Check sheet for the modelled part. Datum: model origin and axes. Units: mm. Face numbers are marked on the shaded views. A direction names the side the tool comes from. Round coordinates to 2 decimals unless told otherwise and drop trailing zeros. Order: outer loops, then holes, each group sorted by start corner. A loop starts at its lowest first (then second) coordinate and runs counter-clockwise, first axis right, second up. Notation, with made-up numbers: (-8.75, 69.25) -> (29.25, 69.25) arc R19 ccw to (29.25, 74.25) -> close; hole circle Ø2 at (83, 82.25). An arc over 180 degrees is marked (long way). Use CSV: the item, a comma, the result in double quotes.
```python
from build123d import *

# Parameters (mm, degrees)
MODEL_R             = 1.25
BOSS_EXTRUDE1_DEPTH = 2


with BuildPart() as part:
    # Model → Boss-Extrude1 (new body)
    with BuildSketch(Plane.XY):
        with BuildLine():
            Line((1953.676808721, 1458.884115951), (1951.176808721, 1458.884115951))
            Line((1951.176808721, 1458.884115951), (1951.176808721, 1462.134115951))
            ThreePointArc((1951.176808721, 1462.134115951), (1956.676808721, 1464.884115951), (1962.176808721, 1462.134115951))
            Line((1962.176808721, 1462.134115951), (1962.176808721, 1458.884115951))
            Line((1962.176808721, 1458.884115951), (1959.676808721, 1458.884115951))
            Line((1959.676808721, 1458.884115951), (1959.676808721, 1456.884115951))
            Line((1959.676808721, 1456.884115951), (1953.676808721, 1456.884115951))
            Line((1953.676808721, 1456.884115951), (1953.676808721, 1458.884115951))
        make_face()
        with Locations((1959.176808721, 1460.884115951)):
            Circle(MODEL_R, mode=Mode.SUBTRACT)
        with Locations((1954.176808721, 1460.884115951)):
            Circle(MODEL_R, mode=Mode.SUBTRACT)
    extrude(amount=BOSS_EXTRUDE1_DEPTH)


solid = part.part
```
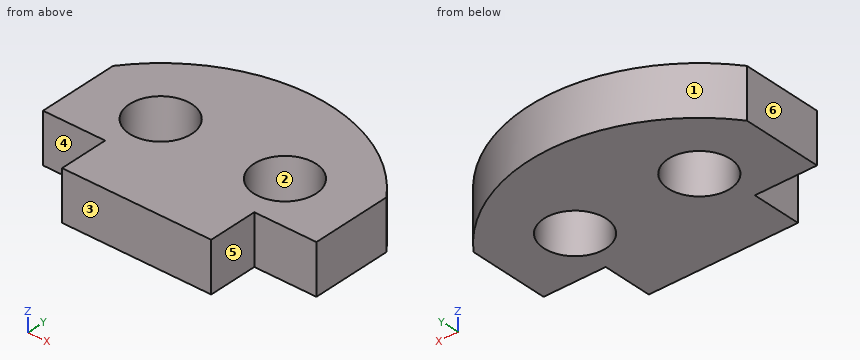
Q1. Go/stop test with flat-tipped pins: pin 1 (1.5 mm diameter, centred on x = 1954.18, y = 1460.88, fed in from +Z); pin 2 (0.6 mm diameter, centred on x = 1952, z = 0.5, fed in from -Y); pin 3 (1 mm diameter, centred on y = 1458, z = 1, fed in from -X). Record where each tip stops, or that it passes through.
Result sheet:
pin 1,"passes through"
pin 2,"stops at y = 1458.88"
pin 3,"stops at x = 1953.68"
Q2. Sectioned sample at C-C, the plane z = 1. Enter the section's corners in (x, y) (3 decimals).
Result sheet:
outline,"(1951.177, 1458.884) -> (1953.677, 1458.884) -> (1953.677, 1456.884) -> (1959.677, 1456.884) -> (1959.677, 1458.884) -> (1962.177, 1458.884) -> (1962.177, 1462.134) arc R6.875 ccw to (1951.177, 1462.134) -> close; hole circle Ø2.5 at (1954.177, 1460.884); hole circle Ø2.5 at (1959.177, 1460.884)"
Q3. Mould release check, pull along Y, two halves, no side actions. Record for the marked faces 1, 2 and 3: pulls with the +Y half, pulls with the -Y half, needs draft (parallel to the pull), parting line crosses it, or undercut.
Result sheet:
face 1,"pulls with the +Y half"
face 2,"undercut"
face 3,"pulls with the -Y half"
Q4. Sectioned sample at B-B, the plane y = 1462. Enter the section's corners in (x, z).
Result sheet:
outline,"(1951.18, 0) -> (1953.61, 0) -> (1953.61, 2) -> (1951.18, 2) -> close; (1954.74, 0) -> (1958.61, 0) -> (1958.61, 2) -> (1954.74, 2) -> close; (1959.74, 0) -> (1962.18, 0) -> (1962.18, 2) -> (1959.74, 2) -> close"
Q5. Sectioned sample at D-D, the plane y = 1458. Enter the section's corners in (x, z), then the cut area to 3 significant figures.
Result sheet:
outline,"(1953.68, 0) -> (1959.68, 0) -> (1959.68, 2) -> (1953.68, 2) -> close"
area,"12.0 mm^2"
Q6. Scan lines: L1, parallel to X at y = 1460, z = 0.65; L2, parallel to X at y = 1460.25, z = 1.3; L3, parallel to Y at x = 1954, z = 1.35. Record each from-to range of solid material in increasing order.
Result sheet:
L1,"x = 1951.18 to 1953.29, 1955.06 to 1958.29, 1960.06 to 1962.18"
L2,"x = 1951.18 to 1953.1, 1955.25 to 1958.1, 1960.25 to 1962.18"
L3,"y = 1456.88 to 1459.65, 1462.12 to 1464.34"
Q7. Access from +Z, -Z, +X, -X, +Y, -Y to the whole of each face (thin tool, end or side, straight path). Record for the marked faces 4, 5 and 6.
Result sheet:
face 4,"+Z, -Z, -X, -Y"
face 5,"+Z, -Z, +X, -Y"
face 6,"+Z, -Z, -X, +Y, -Y"
Q8. Sectioned sample at A-A, the plane x = 1954.5. Enter the section's corners in (y, z), then the cut area to 3 significant figures.
Result sheet:
outline,"(1456.88, 0) -> (1459.68, 0) -> (1459.68, 2) -> (1456.88, 2) -> close; (1462.09, 0) -> (1464.53, 0) -> (1464.53, 2) -> (1462.09, 2) -> close"
area,"10.5 mm^2"
